Autodesk Inventor part; units mm, degrees
ref_plane "YZ Plane" through (0, 0, 0) normal (1, 0, 0) x (0, 1, 0)
ref_plane "XZ Plane" through (0, 0, 0) normal (0, 1, 0) x (-1, 0, 0)
ref_plane "XY Plane" through (0, 0, 0) normal (0, 0, 1) x (1, 0, 0)
sketch "Skizze1" plane through (0, 0, 0) normal (0, 0, 1) x (1, 0, 0)
  line L0 (-28.5, 23) -> (28.5, 23)
  line L1 (28.5, 23) -> (28.5, -23)
  line L2 (28.5, -23) -> (-28.5, -23)
  line L3 (-28.5, -23) -> (-28.5, 23)
  line L4 (0, 32.2) -> (0, -32.2)
  line L5 (-39.9, 0) -> (39.9, 0)
  point P0 (0, 0)
  point P1 (0, 23)
  point P2 (-28.5, 0)
  dimension "d0" = 57
  dimension "d1" = 46
extrude "Extrusion1" add sketch "Skizze1" along normal blind 2
sketch "Skizze2" plane through (0, 0, 0) normal (0, 0, -1) x (-1, 0, 0)
  circle A0 centre (25, -19.5) radius 3.5
  circle A1 centre (-25, -19.5) radius 3.5
  circle A2 centre (25, 19.5) radius 3.5
  circle A3 centre (-25, 19.5) radius 3.5
  line L0 (28.5, -23) -> (-28.5, -23)
  line L1 (28.5, 23) -> (28.5, -23)
  line L2 (-28.5, -23) -> (-28.5, 23)
  line L3 (-28.5, 23) -> (28.5, 23)
  point P0 (0, 0)
  dimension "d4" = 7
  dimension "d5" = 7
  dimension "d6" = 7
  dimension "d7" = 7
  dimension "d8" = 3.5
  dimension "d9" = 3.5
  dimension "d10" = 3.5
  dimension "d11" = 3.5
  dimension "d12" = 3.5
  dimension "d13" = 3.5
  dimension "d14" = 3.5
  dimension "d15" = 3.5
extrude "Extrusion2" add sketch "Skizze2" along normal blind 18 contours A0 | A2 | A1 | A3
sketch "Skizze3" plane through (0, 0, 2) normal (0, 0, 1) x (1, 0, 0)
  circle A0 centre (-25, 19.5) radius 2.75
  circle A1 centre (25, 19.5) radius 2.75
  circle A2 centre (-25, -19.5) radius 2.75
  circle A3 centre (25, -19.5) radius 2.75
  line L0 (28.5, 23) -> (-28.5, 23)
  line L1 (-28.5, 23) -> (-28.5, -23)
  line L2 (28.5, -23) -> (28.5, 23)
  line L3 (-28.5, -23) -> (28.5, -23)
  point P0 (0, 0)
  dimension "d18" = 5.5
  dimension "d19" = 5.5
  dimension "d20" = 5.5
  dimension "d21" = 5.5
  dimension "d22" = 3.5
  dimension "d23" = 3.5
  dimension "d24" = 3.5
  dimension "d25" = 3.5
  dimension "d26" = 3.5
  dimension "d27" = 3.5
  dimension "d28" = 3.5
  dimension "d29" = 3.5
extrude "Extrusion3" cut sketch "Skizze3" against normal blind 4 contours A0 | A1 | A2 | A3
sketch "Skizze4" plane through (-25, 19.5, -2) normal (0, 0, 1) x (1, 0, 0)
  circle A0 centre (0, 0) radius 2.75
  circle A1 centre (0, 0) radius 1.6
  circle A2 centre (50, 0) radius 2.75
  circle A3 centre (50, 0) radius 1.6
  circle A4 centre (50, -39) radius 2.75
  circle A5 centre (50, -39) radius 1.6
  circle A6 centre (0, -39) radius 2.75
  circle A7 centre (0, -39) radius 1.6
  point P0 (25, -19.5)
  dimension "d32" = 3.2
  dimension "d33" = 3.2
  dimension "d34" = 3.2
  dimension "d35" = 3.2
extrude "Extrusion4" cut sketch "Skizze4" against normal up to surface (16 mm away) contours A1 | A3 | A5 | A7
sketch "Skizze5" plane through (-28.5, -23, 2) normal (-1, 0, 0) x (0, 0, 1)
  line L0 (-2, 0) -> (0, 0)
  line L1 (0, 0) -> (-2, 0)
  line L2 (-2, 0) -> (-2, 46)
  line L3 (-2, 46) -> (0, 46)
  line L4 (0, 46) -> (0, 0)
  point P0 (-2, 23)
extrude "Extrusion5" add sketch "Skizze5" along normal blind 15
sketch "Skizze7" plane through (0, 0, 0) normal (0, 0, -1) x (-1, 0, 0)
  circle A0 centre (38.5, -19.5) radius 3.5
  line L0 (25, -23) -> (43.5, -23)
  line L1 (43.5, 23) -> (43.5, -23)
  circle A1 centre (38.5, 19.5) radius 3.5
  line L2 (25, 23) -> (43.5, 23)
  circle A2 centre (-17.5, 19.5) radius 3.5
  line L3 (-25, 23) -> (25, 23)
  line L4 (-28.5, -19.5) -> (-28.5, 19.5)
  circle A3 centre (-17.5, -19.5) radius 3.5
  line L5 (25, -23) -> (-25, -23)
  line L6 (-28.5, -23) -> (-28.5, -19.5)
  point P0 (0, 0)
  dimension "d53" = 7
  dimension "d54" = 3.5
  dimension "d55" = 5
  dimension "d56" = 7
  dimension "d57" = 5
  dimension "d58" = 3.5
  dimension "d59" = 7
  dimension "d60" = 3.5
  dimension "d61" = 11
  dimension "d62" = 7
  dimension "d63" = 3.5
  dimension "d64" = 11
extrude "Extrusion6" add sketch "Skizze7" along normal blind 5
sketch "Skizze6" plane through (0, 0, 2) normal (0, 0, 1) x (1, 0, 0)
  circle A0 centre (17.5, -19.5) radius 2.25
  circle A1 centre (17.5, 19.5) radius 2.25
  circle A2 centre (-38.5, -19.5) radius 2.25
  circle A3 centre (-38.5, 19.5) radius 2.25
  line L0 (-57.9, 0) -> (42.9, 0)
  line L1 (-43.5, -23) -> (-43.5, 23)
  point P0 (0, 0)
  dimension "d40" = 4.5
  dimension "d41" = 4.5
  dimension "d42" = 4.5
  dimension "d43" = 4.5
  dimension "d44" = 39
  dimension "d45" = 39
  dimension "d46" = 19.5
  dimension "d47" = 19.5
  dimension "d48" = 19.5
  dimension "d49" = 19.5
  dimension "d50" = 56
  dimension "d51" = 5
extrude "Extrusion7" cut sketch "Skizze6" against normal blind 6
sketch "Skizze8" plane through (0, 0, 2) normal (0, 0, 1) x (1, 0, 0)
  line L0 (-39.5, 15.5) -> (24.5, 15.5)
  line L1 (24.5, 15.5) -> (24.5, -15.5)
  line L2 (24.5, -15.5) -> (-39.5, -15.5)
  line L3 (-39.5, -15.5) -> (-39.5, 15.5)
  line L4 (28.5, -23) -> (28.5, 23)
  line L5 (28.5, 23) -> (-43.5, 23)
  line L6 (-43.5, -23) -> (-43.5, 23)
  line L7 (28.5, -23) -> (-43.5, -23)
  point P0 (0, 0)
  dimension "d69" = 4
  dimension "d70" = 7.5
  dimension "d71" = 4
  dimension "d72" = 7.5
extrude "Extrusion8" cut sketch "Skizze8" against normal up to surface (2 mm away) contours L0 L1 L2 L3
properties part number "_3D-Druck"
Verification items for the finished model (mm, model axes). A direction names the side the tool comes from. Round coordinates to 2 decimals unless told otherwise and drop trailing zeros. Write each loop counter-clockwise with the first axis right and the second up, starting at its lowest first coordinate (ties: lowest second). Pieces come first, ordered by that corner, then holes.
(1) Section check A-A (z = -13.5). Enter the section's corners in (x, y).
Returned:
outline: circle Ø7 at (-25, -19.5); circle Ø7 at (-25, 19.5); circle Ø7 at (25, -19.5); circle Ø7 at (25, 19.5); hole circle Ø3.2 at (-25, -19.5); hole circle Ø3.2 at (-25, 19.5); hole circle Ø3.2 at (25, -19.5); hole circle Ø3.2 at (25, 19.5)
(2) Section check C-C (y = -8). Enter the section's corners in (x, z).
Returned:
outline: (-43.5, 0) - (-39.5, 0) - (-39.5, 2) - (-43.5, 2) - close; (24.5, 0) - (28.5, 0) - (28.5, 2) - (24.5, 2) - close
(3) Mould release check, pull along Y, two halves, no side actions. Record for faces 1 (the flat face through (-39.5, 0, 1)), 2 (the flat face through (28.5, 0, 1)): pulls with the +Y half, pulls with the -Y half, needs draft (parallel to the pull), parting line crosses it, or undercut.
Returned:
face 1: undercut
face 2: needs draft
(4) Section check B-B (x = 6.5). Enter the section's corners in (y, z).
Returned:
outline: (-23, 0) - (-15.5, 0) - (-15.5, 2) - (-23, 2) - close; (15.5, 0) - (23, 0) - (23, 2) - (15.5, 2) - close
(5) Section check D-D (z = 0.75). Give the number of separate pieces and of enclosed holes in the cut face, plus the area to 3 significant figures.
Returned:
separate pieces: 1
enclosed holes: 9
area: 1,170 mm2
(6) Material ranges on line 1 (Y direction, x = -38.5, z = -1.9); line 2 (Y direction, x = -25, z = 0.8); line 3 (Z direction, x = -40, y = -3.5), recorded low to high.
Returned:
line 1: y = -23 to -21.75, -17.25 to -16, 16 to 17.25, 21.75 to 23
line 2: y = -23 to -22.25, -16.75 to -15.5, 15.5 to 16.75, 22.25 to 23
line 3: z = 0 to 2
(7) Access from +Z, -Z, +X, -X, +Y, -Y to the whole of each face (thin tool, end or side, straight path). Record for faces 3 (the flat face through (28, 22, 0)), 4 (the cylindrical face through (-27.747, 19.621, 0.028)), 5 (the flat face through (24.5, 0, 1)), 6 (the flat face through (18, -19, -5)), 7 (the flat face through (-7, -17, 0)).
Returned:
face 3: -Z, +X, +Y
face 4: +Z
face 5: +Z, -Z
face 6: -Z, +Y, -Y
face 7: -Z
(8) Depth check by flat-ended pin: pin 1 Ø2.5 at (x, y) = (-38.5, -19.5) entering from +Z; pin 2 Ø1.9 at (x, y) = (-25, 19.5) entering from -Z; pin 3 Ø2 at (x, y) = (-40, 18) entering from -Z; pin 4 Ø3 at (x, y) = (26, -19) entering from +Z. Enter the tip coordinate at first touch or a pass-through.
Returned:
pin 1: stops at z = -4
pin 2: passes through
pin 3: stops at z = -5
pin 4: stops at z = -2
